Geometry: see drawing. Coordinates: mm, zero at the bounding-box minimum. A direction names the side the tool comes from. Coordinates: 2 decimals unless noted, no trailing zeros. Order: outer loops, then holes, each group sorted by start corner. A loop starts at its lowest first (then second) coordinate and runs counter-clockwise, first axis right, second up. Notation, with made-up numbers: M 62.5,59.25 L 68.5,59.25 A17 ccw 68.5,88.25 Z; hole C -16,-16.75 d10. An arc over 180 degrees is marked long. One line per item, written item: value.
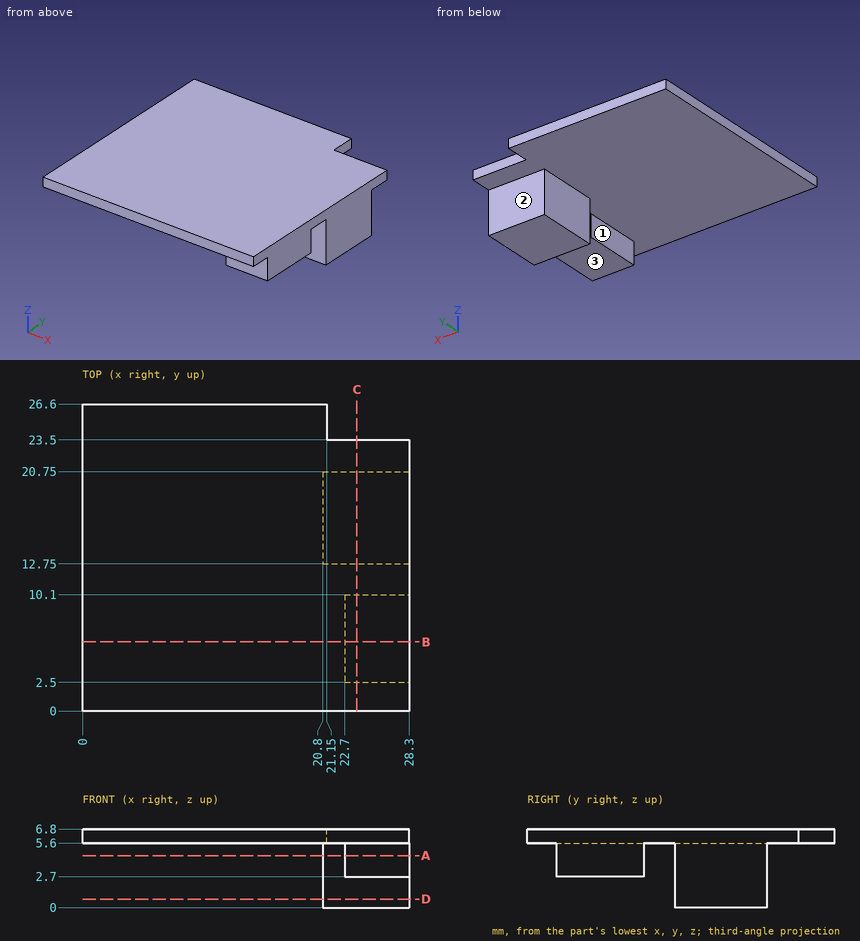
(1) Cut plane B-B on y = 6. Output: boundary loops of the cut face in (x, z), plus the area to 3 significant figures.
Data:
outline: M 0,5.6 L 22.7,5.6 L 22.7,2.7 L 28.3,2.7 L 28.3,6.8 L 0,6.8 Z
area: 50.2 mm2
(2) Cut plane D-D on z = 0.75. Output: boundary loops of the cut face in (x, y).
Data:
outline: M 20.8,12.75 L 28.3,12.75 L 28.3,20.75 L 20.8,20.75 Z
(3) Cut plane C-C on x = 23.75. Output: boundary loops of the cut face in (y, z), plus the area to 3 significant figures.
Data:
outline: M 0,5.6 L 2.5,5.6 L 2.5,2.7 L 10.1,2.7 L 10.1,5.6 L 12.75,5.6 L 12.75,0 L 20.75,0 L 20.75,5.6 L 23.5,5.6 L 23.5,6.8 L 0,6.8 Z
area: 95.0 mm2
(4) Access query for the marked faces 1, 2 and 3. Directions: +Z, -Z, +X, -X, +Y, -Y. A direction counts if a zero-diameter tool reaches every point of the face in a straight line with its end or side. Return the directions, or none.
Data:
face 1: -Z, -X, -Y
face 2: -Z, +X, -X, +Y
face 3: -Z, +X, -X, -Y
(5) First-contact query: pin 1 (2.5 mm diameter, centred on x = 26, z = 5, fed in from -Y); pin 2 (4 mm diameter, centred on x = 17.5, y = 15, fed in from -Z); pin 3 (3 mm diameter, centred on x = 25.5, z = 3.5, fed in from +Y); pin 4 (1 mm diameter, centred on x = 25, z = 6.5, fed in from +Y). Flat tips, straight axial feed; report the tip coordinate or a pass-through.
Data:
pin 1: stops at y = 0
pin 2: stops at z = 5.6
pin 3: stops at y = 20.75
pin 4: stops at y = 23.5
(6) Cut plane A-A on z = 4.5. Output: boundary loops of the cut face in (x, y), plus the area to 3 significant figures.
Data:
outline: M 20.8,12.75 L 28.3,12.75 L 28.3,20.75 L 20.8,20.75 Z; M 22.7,2.5 L 28.3,2.5 L 28.3,10.1 L 22.7,10.1 Z
area: 103 mm2
(7) Ray query, line 1 (Z direction, x = 18.75, y = 4.5); line 2 (X direction, y = 5, z = 2.75); line 3 (X direction, y = 13.75, z = 4). Return the intervals inside material, ascending. Write a range as from..to.
Data:
line 1: z = 5.6..6.8
line 2: x = 22.7..28.3
line 3: x = 20.8..28.3
